Source: CAD feature listing. Evaluate the final solid. Frame: model axes, mm. A direction names the side the tool comes from. Coordinates: 2 decimals unless noted, no trailing zeros. Order: outer loops, then holes, each group sorted by start corner. A loop starts at its lowest first (then second) coordinate and runs counter-clockwise, first axis right, second up.
```python
from build123d import *

# Parameters (mm, degrees)
SKETCH1_W            = 256
SKETCH1_H            = 50
SKETCH1_R            = 2
BOSS_EXTRUDE1_DEPTH  = 8
FILLET1_R            = 4
SKETCH2_W            = 7
SKETCH2_H            = 8
BOSS_EXTRUDE2_DEPTH  = 8
SKETCH3_W            = 50
SKETCH3_H            = 20
CUT_EXTRUDE1_DEPTH   = 8
SKETCH4_R            = 2
CUT_EXTRUDE2_DEPTH   = 8
SKETCH5_R            = 1.75
CUT_EXTRUDE3_DEPTH   = 113
BOSS_EXTRUDE12_START = 7.5
SKETCH8_W            = 200
SKETCH8_H            = 8
BOSS_EXTRUDE12_DEPTH = 10


with BuildPart() as part:
    # Sketch1 → Boss-Extrude1 (new body)
    with BuildSketch(Plane.XY):
        with Locations((0.283809042, 47.106089777)):
            Rectangle(SKETCH1_W, SKETCH1_H)
        with Locations((120.283809042, 65.106089777)):
            Circle(SKETCH1_R, mode=Mode.SUBTRACT)
        with Locations((111.283809042, 65.106089777)):
            Circle(SKETCH1_R, mode=Mode.SUBTRACT)
        with Locations((8.283809042, 65.106089777)):
            Circle(SKETCH1_R, mode=Mode.SUBTRACT)
        with Locations((-7.716190958, 65.106089777)):
            Circle(SKETCH1_R, mode=Mode.SUBTRACT)
        with Locations((-16.716190958, 65.106089777)):
            Circle(SKETCH1_R, mode=Mode.SUBTRACT)
        with Locations((-119.716190958, 65.106089777)):
            Circle(SKETCH1_R, mode=Mode.SUBTRACT)
    extrude(amount=BOSS_EXTRUDE1_DEPTH)

    # Fillet1
    fillet1_edges = [part.edges().sort_by_distance(p)[0] for p in [
        (-127.716190958, 72.106089777, 4),
        (128.283809042, 72.106089777, 4),
        (128.283809042, 22.106089777, 4),
        (-127.716190958, 22.106089777, 4),
    ]]
    fillet(fillet1_edges, radius=FILLET1_R)

    # Sketch2 → Boss-Extrude2 (add)
    with BuildSketch(Plane.XY.offset(8)):
        with Locations((36.783809042, 18.106089777)):
            Rectangle(SKETCH2_W, SKETCH2_H)
        with Locations((-36.216190958, 18.106089777)):
            Rectangle(SKETCH2_W, SKETCH2_H)
    extrude(amount=-BOSS_EXTRUDE2_DEPTH)

    # Sketch3 → Cut-Extrude1 (cut)
    with BuildSketch(Plane.XY.offset(8)):
        with Locations((0.283809042, 32.106089777)):
            Rectangle(SKETCH3_W, SKETCH3_H)
    extrude(amount=-CUT_EXTRUDE1_DEPTH, mode=Mode.SUBTRACT)

    # Sketch4 → Cut-Extrude2 (cut)
    with BuildSketch(Plane.XY.offset(8)):
        with Locations((-31.716190958, 32.106089777)):
            Circle(SKETCH4_R)
        with Locations((32.283809042, 32.106089777)):
            Circle(SKETCH4_R)
        with Locations((-119.716190958, 32.106089777)):
            Circle(SKETCH4_R)
        with Locations((120.283809042, 29.106089777)):
            Circle(SKETCH4_R)
    extrude(amount=-CUT_EXTRUDE2_DEPTH, mode=Mode.SUBTRACT)

    # Sketch5 → Cut-Extrude3 (cut)
    with BuildSketch(Plane.ZY.offset(39.716190958)):
        with Locations((3.5, 18.106089777)):
            Circle(SKETCH5_R)
    extrude(amount=-CUT_EXTRUDE3_DEPTH, mode=Mode.SUBTRACT)

    # Sketch8 → Boss-Extrude12 (add)
    with BuildSketch(Plane.XY.offset(BOSS_EXTRUDE12_START)):
        with Locations((0.283809042, 18.106089777)):
            Rectangle(SKETCH8_W, SKETCH8_H)
    extrude(amount=BOSS_EXTRUDE12_DEPTH)


solid = part.part
```
1. Pin query (flat end, axial travel): P1, Ø12, axis at x = 5, y = 50, coming from the +Z side; P2, Ø2.5, axis at x = 77.5, y = 18, coming from the -Z side; P3, Ø4, axis at x = 101.5, z = 4.5, coming from the -Y side. Return the tip coordinate at first contact, or that it passes through.
Findings:
P1: stops at z = 8
P2: stops at z = 7.5
P3: stops at y = 22.11
2. Section query A-A on x = -37. Return loops of the section in (y, z).
Findings:
outline: (14.11, 0) - (72.11, 0) - (72.11, 8) - (22.11, 8) - (22.11, 17.5) - (14.11, 17.5) - close; hole circle Ø3.5 at (18.11, 3.5)
3. Draft query along Y for faces 1 (the face through (-1, 14.106, 13)), 2 (the face through (127.081, 70.965, 4.056)), 3 (the face through (100.284, 18, 12)), 4 (the face through (119.85, 63.154, 3.944)). Return one class per face: released by +Y, released by -Y, zero draft, split by the parting line, or undercut.
Findings:
face 1: released by -Y
face 2: released by +Y
face 3: zero draft
face 4: undercut
4. Ray query, line 1 (X direction, y = 39, z = 7); line 2 (Z direction, x = -76.5, y = 36); line 3 (Y direction, x = 78, z = 14.5). Return the intervals inside material, ascending.
Findings:
line 1: x = -127.72 to -24.72, 25.28 to 128.28
line 2: z = 0 to 8
line 3: y = 14.11 to 22.11
5. Access query for faces 5 (the face through (-1, 18, 17.5)), 6 (the face through (0, 18, 7.5)), 7 (the face through (-39.716, 18.1, 5.5)). Directions: +Z, -Z, +X, -X, +Y, -Y. A direction counts if a zero-diameter tool reaches every point of the face in a straight line with its end or side. Return the directions, or none.
Findings:
face 5: +Z, +X, -X, +Y, -Y
face 6: -Z, -Y
face 7: -Z, -X, -Y
